Build history of the part. All positions in model axes, mm. A direction names the side the tool comes from. Round coordinates to 2 decimals unless told otherwise and drop trailing zeros. Loops run counter-clockwise (first coordinate to the right, second up) from the corner with the lowest first, then second, coordinate; pieces in that order, holes last. Notation, with made-up numbers: (-17.5, -30.5) - (37.5, -30.5) arc R17 ccw to (37.5, -2.5) - close; hole circle Ø5 at (11.25, 35). An arc over 180 degrees is marked (long way). One line per question, with ' | ' between items. Start each with the question number.
Autodesk Inventor part; units mm, degrees
ref_plane "YZ Plane" through (0, 0, 0) normal (1, 0, 0) x (0, 1, 0)
ref_plane "XZ Plane" through (0, 0, 0) normal (0, 1, 0) x (-1, 0, 0)
ref_plane "XY Plane" through (0, 0, 0) normal (0, 0, 1) x (1, 0, 0)
sketch "スケッチ1" plane through (0, 0, 0) normal (1, 0, 0) x (0, 1, 0)
  circle A0 centre (0, 0) radius 20
  circle A1 centre (0, 0) radius 9.75
  line L0 (0, 0) -> (35.25, 0)
  line L1 (35.25, 0) -> (35.25, -14.25)
  line L2 (35.25, -14.25) -> (0, -14.25)
  line L3 (0, -14.25) -> (0, 0)
  line L4 (35.25, 0) -> (35.25, 14.25)
  line L5 (35.25, 14.25) -> (0, 14.25)
  point P0 (14.0334, 14.25)
  point P1 (14.0334, -14.25)
  dimension "d0" = 40
  dimension "d1" = 19.5
  dimension "d2" = 14.25
  dimension "d3" = 35.25
extrude "押し出し1" add sketch "スケッチ1" along normal blind 3
sketch "スケッチ2" plane through (0, 0, 0) normal (-1, 0, 0) x (0, 0, 1)
  arc A0 (-14.25, 14.0334) -> (14.25, 14.0334) centre (0, 0) ccw
  circle A1 centre (0, 0) radius 9.75
  dimension "d6" = 19.5
extrude "押し出し2" cut sketch "スケッチ2" against normal blind 2.1
sketch "スケッチ3" plane through (2.1, 0, 0) normal (-1, 0, 0) x (0, 0, 1)
  circle A0 centre (0, 0) radius 8
  point P0 (0, 8)
  point P1 (-5.6569, 5.6569)
  point P2 (-8, 0)
  point P3 (-5.6569, -5.6569)
  point P4 (0, -8)
  point P5 (5.6569, -5.6569)
  point P6 (8, 0)
  point P7 (5.6569, 5.6569)
  dimension "d9" = 16
  dimension "d12" = 360
hole "穴1" at (2.1, 8, 0) at (2.1, 5.6569, -5.6569) at (2.1, 0, -8) at (2.1, -5.6569, -5.6569) at (2.1, -8, 0) at (2.1, -5.6569, 5.6569) at (2.1, 0, 8) at (2.1, 5.6569, 5.6569) direction (1, 0, 0) diameter 2.1 end through all
sketch "スケッチ4" plane through (3, 0, 0) normal (1, 0, 0) x (0, 0, -1)
  line L0 (-14.25, 35.25) -> (-14.25, 14.0334)
  line L1 (-14.25, 35.25) -> (14.25, 35.25)
  line L2 (14.25, 35.25) -> (14.25, -11.25)
  line L3 (14.25, -11.25) -> (-14.25, -11.25)
  line L4 (-14.25, -11.25) -> (-14.25, 35.25)
  point P0 (0, 0)
  point P1 (-11, -8)
  point P2 (11, -8)
  point P3 (-11, 32)
  point P4 (11, 32)
  dimension "d21" = 46.5
  dimension "d22" = 3.25
  dimension "d23" = 3.25
  dimension "d24" = 3.25
  dimension "d25" = 3.25
  dimension "d26" = 3.25
  dimension "d27" = 3.25
  dimension "d28" = 3.25
  dimension "d29" = 3.25
hole "穴2" at (3, -8, 11) at (3, -8, -11) at (3, 32, -11) at (3, 32, 11) direction (-1, 0, 0) diameter 2.5 end through all
sketch "スケッチ5" plane through (0, 0, 0) normal (-1, 0, 0) x (0, 0, 1)
  circle A0 centre (-11, -8) radius 1.25
  circle A1 centre (-11, -8) radius 2.4
  circle A2 centre (11, -8) radius 1.25
  circle A3 centre (11, -8) radius 2.4
  circle A4 centre (-11, 32) radius 1.25
  circle A5 centre (-11, 32) radius 2.4
  circle A6 centre (11, 32) radius 1.25
  circle A7 centre (11, 32) radius 2.4
  point P0 (0, 0)
  dimension "d37" = 4.8
  dimension "d38" = 4.8
  dimension "d39" = 4.8
  dimension "d40" = 4.8
extrude "押し出し3" cut sketch "スケッチ5" against normal blind 2.5 contours A1 | A2 | A3 | A4 | A5 | A6 | A7
fillet "フィレット1" radius 3 4 edges at (1.5, 35.25, -14.25) (1.5, 35.25, 14.25) (1.5, 14.0334, -14.25) (1.5, 14.0334, 14.25)
sketch "スケッチ6" plane through (2.1, 0, 0) normal (-1, 0, 0) x (0, 0, 1)
  circle A0 centre (0, 0) radius 4.05
  dimension "d44" = 8.1
extrude "押し出し4" cut sketch "スケッチ6" against normal blind 10
properties part number "connectplate3" material "アルミニウム 6061"
1) Saw through at B-B on y = 0. Write the cut outline in (x, z).
2) Saw through at D-D on z = 8. Write the cut outline in (x, y).
3) Drop flat-ended pins along their axis: pin 1 (1.4 mm diameter, centred on y = -7.5, z = -10.5, fed in from -X); pin 2 (1 mm diameter, centred on x = 2.5, y = -6.5, fed in from -Z); pin 3 (3.5 mm diameter, centred on y = 5.66, z = 5.66, fed in from +X); pin 4 (1.5 mm diameter, centred on x = 1, y = -7.5, fed in from +Z). Give the stop position or say it passes through.
4) Tool access for faces 1 (the cylindrical face through (2.75, -8.05, 12.25)), 2 (the flat face through (2.1, 0.1, 4.2)), 3 (the flat face through (1, 24, 14.25)): list every direction of +Z, -Z, +X, -X, +Y, -Y with a clear straight run to the whole face (end or side of a thin tool).
5) Two-plate mould, pull along Z, no slides. Class faces 4 (the cylindrical face through (2.556, 6.296, 4.824)), 5 (the flat face through (0, 13, 0)), 6 (the flat face through (1, 24, -14.25)): +Z half, -Z half, draft (parallel to the pull), parting line (faces both ways), or undercut.
6) Saw through at A-A on z = 0. Write the cut outline in (x, y), and give its area (3 significant figures).
7) Saw through at C-C on y = 8. Write the cut outline in (x, z).
8) Wall check: line 1 (Y direction, x = 2.6, z = 0); line 2 (Y direction, x = 2.6, z = 10); line 3 (Z direction, x = 1.5, y = 0.5). Give the ranges that are in metal, low to high. Write a range as [from, to].
Answer key:
1) outline: (0, -20) - (3, -20) - (3, -9.05) - (2.1, -9.05) - (2.1, -9.75) - (0, -9.75) - close; (0, 9.75) - (2.1, 9.75) - (2.1, 9.05) - (3, 9.05) - (3, 20) - (0, 20) - close; (2.1, -6.95) - (3, -6.95) - (3, -4.05) - (2.1, -4.05) - close; (2.1, 4.05) - (3, 4.05) - (3, 6.95) - (2.1, 6.95) - close
2) outline: (0, -18.33) - (3, -18.33) - (3, -1.05) - (2.1, -1.05) - (2.1, -5.57) - (0, -5.57) - close; (0, 5.57) - (2.1, 5.57) - (2.1, 1.05) - (3, 1.05) - (3, 35.25) - (0, 35.25) - close
3) pin 1: x = 2.5 | pin 2: z = -19.08 | pin 3: x = 3 | pin 4: z = 18.83
4) face 1: +X, -X | face 2: -X | face 3: +Z, +X, -X, +Y
5) face 4: undercut | face 5: draft | face 6: -Z half
6) outline: (0, -20) - (3, -20) - (3, -9.05) - (2.1, -9.05) - (2.1, -9.75) - (0, -9.75) - close; (0, 9.75) - (2.1, 9.75) - (2.1, 9.05) - (3, 9.05) - (3, 35.25) - (0, 35.25) - close; (2.1, -6.95) - (3, -6.95) - (3, -4.05) - (2.1, -4.05) - close; (2.1, 4.05) - (3, 4.05) - (3, 6.95) - (2.1, 6.95) - close | area: 114 mm²
7) outline: (0, -18.33) - (3, -18.33) - (3, -1.05) - (2.1, -1.05) - (2.1, -5.57) - (0, -5.57) - close; (0, 5.57) - (2.1, 5.57) - (2.1, 1.05) - (3, 1.05) - (3, 18.33) - (0, 18.33) - close
8) line 1: [-20, -9.05], [-6.95, -4.05], [4.05, 6.95], [9.05, 35.25] | line 2: [-17.32, -8.75], [-7.25, 31.25], [32.75, 35.25] | line 3: [-19.99, -9.74], [9.74, 19.99]
